Check sheet for the modelled part. Datum: model origin and axes. Units: mm. A direction names the side the tool comes from. Give positions to 0.01 mm unless a question says otherwise; leave off trailing zeros. Order: outer loops, then holes, each group sorted by start corner. A loop starts at its lowest first (then second) coordinate and runs counter-clockwise, first axis right, second up.
```python
from build123d import *

# Parameters (mm, degrees)
PAD005_DEPTH      = 0.6
PAD005_DEPTH_BACK = 5
FILLET004_R       = 0.4
THICKNESS_T       = -0.2


with BuildPart() as part:
    # Sketch007 (on Face1 of ReferenceLinearPattern004001) → Pad005 (new body, two sides)
    with BuildSketch(Plane.XZ) as pad005_sk:
        with BuildLine():
            Line((44.9, 2.7), (38, 2.7))
            ThreePointArc((38, 2.7), (37.787868, 2.612132), (37.7, 2.4))
            Line((37.7, 1.8), (37.7, 2.4))
            Line((38.2, 1), (37.7, 1.8))
            Line((38.2, 1), (44.7, 1))
            Line((44.7, 1), (45.2, 1.8))
            Line((45.2, 1.8), (45.2, 2.4))
            ThreePointArc((45.2, 2.4), (45.112132, 2.612132), (44.9, 2.7))
        make_face()
    extrude(amount=PAD005_DEPTH)
    extrude(pad005_sk.sketch, amount=-PAD005_DEPTH_BACK)

    # Fillet004
    fillet004_edges = [part.edges().sort_by_distance(p)[0] for p in [
        (37.7, 2.2, 1.8),
        (38.2, 2.2, 1),
        (45.2, 2.2, 1.8),
        (44.7, 2.2, 1),
    ]]
    fillet(fillet004_edges, radius=FILLET004_R)

    # Thickness
    thickness_openings = [part.faces().sort_by_distance(p)[0] for p in [
        (41.45, -0.6, 1.867545),
    ]]
    offset(amount=THICKNESS_T, openings=thickness_openings)


solid = part.part
```
(1) Release check for a two-part mould opening along X. For faces 3 (the face through (41, 2, 2.7)), 4 (the face through (41, 2, 2.5)) record: released by +X, released by -X, zero draft, split by the parting line, or undercut.
Response values:
face 3: zero draft
face 4: undercut
(2) Set-up check for faces 1 (the face through (41, 2, 1)), 2 (the face through (41, 4.8, 2)): record each of +Z, -Z, +X, -X, +Y, -Y from which the full face is reachable in a straight line by a thin tool's end or side.
Response values:
face 1: -Z, +X, -X, +Y, -Y
face 2: -Y
(3) Cross-section at D-D on z = 1.1. Enter the section's corners in (x, y), then the cut area to 3 significant figures.
Response values:
outline: (38.16, -0.6) - (44.74, -0.6) - (44.74, 5) - (38.16, 5) - close
area: 36.9 mm2
(4) Cross-section at B-B on y = 2.7. Enter the section's corners in (x, z), then the cut area to 3 significant figures.
Response values:
outline: (37.7, 1.91) arc R0.4 ccw to (37.76, 1.7) - (38.08, 1.19) arc R0.4 ccw to (38.42, 1) - (44.48, 1) arc R0.4 ccw to (44.82, 1.19) - (45.14, 1.7) arc R0.4 ccw to (45.2, 1.91) - (45.2, 2.4) arc R0.3 ccw to (44.9, 2.7) - (38, 2.7) arc R0.3 ccw to (37.7, 2.4) - close; hole (37.9, 1.91) arc R0.2 ccw to (37.93, 1.81) - (38.25, 1.29) arc R0.2 ccw to (38.42, 1.2) - (44.48, 1.2) arc R0.2 ccw to (44.65, 1.29) - (44.97, 1.81) arc R0.2 ccw to (45, 1.91) - (45, 2.4) arc R0.1 ccw to (44.9, 2.5) - (38, 2.5) arc R0.1 ccw to (37.9, 2.4) - close
area: 3.34 mm2
(5) Material ranges on L1, parallel to X at y = 2.3, z = 2.05; L2, parallel to Z at x = 42, y = 0.7; L3, parallel to Y at x = 39.25, z = 1.45, recorded low to high.
Response values:
L1: x = 37.7 to 37.9, 45 to 45.2
L2: z = 1 to 1.2, 2.5 to 2.7
L3: y = 4.8 to 5
(6) Cross-section at C-C on x = 44. Enter the section's corners in (y, z).
Response values:
outline: (-0.6, 1) - (5, 1) - (5, 2.7) - (-0.6, 2.7) - (-0.6, 2.5) - (4.8, 2.5) - (4.8, 1.2) - (-0.6, 1.2) - close
(7) Gauge pin test, flat end, axial feed: pin 1 Ø0.7 at (x, z) = (42, 2) entering from -Y. Record the tip position at first contact, or that the pin passes through.
Response values:
pin 1: stops at y = 4.8
(8) Cross-section at A-A on z = 2.25. Enter the section's corners in (x, y).
Response values:
outline: (37.7, -0.6) - (37.9, -0.6) - (37.9, 4.8) - (45, 4.8) - (45, -0.6) - (45.2, -0.6) - (45.2, 5) - (37.7, 5) - close
